For this review, take the finished solid that the model builds, in its own axes (mm). Coordinates: 2 decimals unless noted, no trailing zeros. Loops run counter-clockwise (first coordinate to the right, second up) from the corner with the lowest first, then second, coordinate; pieces in that order, holes last. Notation, with made-up numbers: M 12,64.25 L 45,64.25 A22 cw 45,75.25 Z; hole C 60,-6.5 d2. An arc over 180 degrees is marked long. Write item = value, one per line.
from build123d import *

# Parameters (mm, degrees)
SKETCH1_R           = 175
BOSS_EXTRUDE1_DEPTH = 400
SCALE1_SCALE        = 0.1
SKETCH3_R           = 3
CUT_EXTRUDE1_DEPTH  = 41


with BuildPart() as part:
    # Sketch1 → Boss-Extrude1 (new body)
    with BuildSketch(Plane(origin=(0, 0, 0), x_dir=(1, 0, 0), z_dir=(0, 1, 0))):
        Circle(SKETCH1_R)
    extrude(amount=BOSS_EXTRUDE1_DEPTH)


with BuildPart() as part_1:
    # Scale1: scaled about (0, 200, 0)
    add(part.part.scale(SCALE1_SCALE).moved(Location((0, 180, 0))))

    # Sketch3 → Cut-Extrude1 (cut, through all)
    with BuildSketch(Plane(origin=(0, 220, 0), x_dir=(1, 0, 0), z_dir=(0, 1, 0))):
        Circle(SKETCH3_R)
    extrude(amount=-CUT_EXTRUDE1_DEPTH, mode=Mode.SUBTRACT)


solid = part_1.part
Q1. Add section A-A (x = 0). Write out the cut boundary in (y, z), and give its area (3 significant figures).
Solved:
outline = M 180,-17.5 L 220,-17.5 L 220,-3 L 180,-3 Z; M 180,3 L 220,3 L 220,17.5 L 180,17.5 Z
area = 1,160 mm²
Q2. Draft analysis for pull direction X (two halves, no side actions). For faces 1 (the face through (-13.887, 199.72, 10.648)), 2 (the face through (-3, 200, 0)), 3 (the face through (0, 180, 4)), state which applies: +X half, -X half, draft (parallel to the pull), parting line (faces both ways), or undercut.
Solved:
face_1 = parting line
face_2 = undercut
face_3 = draft
Q3. For line 1 along Z through (x, y) = (0, 207.5); line 2 along Z through (x, y) = (-6, 203), list the stretches that pass through material, from the lowest coordinate up.
Solved:
line_1 = -17.5 to -3, 3 to 17.5
line_2 = -16.44 to 16.44
Q4. Add section D-D (x = -10.5). Write out the cut boundary in (y, z).
Solved:
outline = M 180,-14 L 220,-14 L 220,14 L 180,14 Z
Q5. Add section B-B (z = 0). Write out the cut boundary in (x, y).
Solved:
outline = M -17.5,180 L -3,180 L -3,220 L -17.5,220 Z; M 3,180 L 17.5,180 L 17.5,220 L 3,220 Z
Q6. For pin 1 Ø3.5 at (x, z) = (0, 0) entering from -Y; pin 2 Ø5 at (x, y) = (-11, 185.5) entering from -Z; pin 3 Ø12 at (y, z) = (204, -11) entering from -X; pin 4 Ø5 at (y, z) = (196, -9) entering from +X, all flat-tipped, find the tip position at first contact; note any pin that passes through.
Solved:
pin_1 = through
pin_2 = -15.3
pin_3 = -16.77
pin_4 = 16.25
Q7. Add section C-C (y = 204). Write out the cut boundary in (x, z), and give its area (3 significant figures).
Solved:
outline = C 0,0 d35; hole C 0,0 d6
area = 934 mm²
